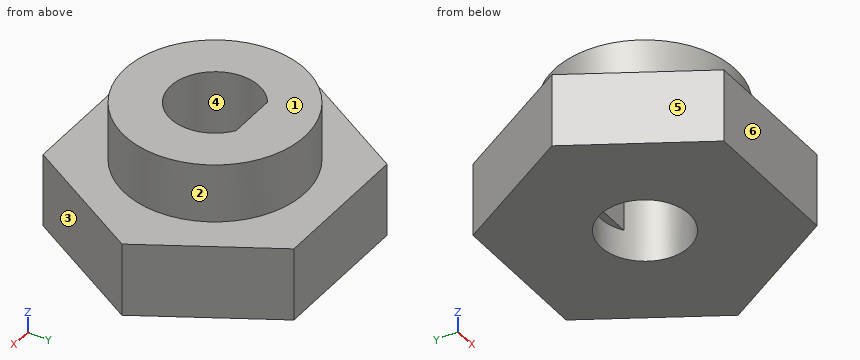
```python
from build123d import *

# Parameters (mm, degrees)
SKETCH_R      = 3
PAD_DEPTH     = 5
SKETCH001_R   = 6.1
SKETCH001_R_2 = 3
PAD001_DEPTH  = 10
PAD002_DEPTH  = 13
SKETCH003_R   = 6.1
POCKET_DEPTH  = 6


with BuildPart() as part:
    # Sketch → Pad (new body)
    with BuildSketch(Plane.XY):
        Polygon((9.814955, 0), (4.907477, 8.5), (-4.907477, 8.5), (-9.814955, 0), (-4.907477, -8.5), (4.907477, -8.5), align=None)
        Circle(SKETCH_R, mode=Mode.SUBTRACT)
    extrude(amount=PAD_DEPTH)

    # Sketch001 (on Face9 of Pad) → Pad001 (join)
    with BuildSketch(Plane.XY.offset(5)):
        Circle(SKETCH001_R)
        Circle(SKETCH001_R_2, mode=Mode.SUBTRACT)
    extrude(amount=PAD001_DEPTH)

    # Sketch002 (on Face12 of Pad001) → Pad002 (join)
    with BuildSketch(Plane.XY.offset(15)):
        with BuildLine():
            Line((-1.658312, 2.5), (1.658312, 2.5))
            ThreePointArc((1.658312, 2.5), (0, 3), (-1.658312, 2.5))
        make_face()
    extrude(amount=-PAD002_DEPTH)

    # Sketch003 (on Face15 of Pad002) → Pocket (cut)
    with BuildSketch(Plane.XY.offset(15)):
        Circle(SKETCH003_R)
    extrude(amount=-POCKET_DEPTH, mode=Mode.SUBTRACT)


solid = part.part
```
For this review, take the finished solid that the model builds, in its own axes (mm). Face numbers are marked on the shaded views. A direction names the side the tool comes from. Round coordinates to 2 decimals unless told otherwise and drop trailing zeros. Order: outer loops, then holes, each group sorted by start corner. A loop starts at its lowest first (then second) coordinate and runs counter-clockwise, first axis right, second up.
Q1. We need section D-D, the plane z = 1.5. Give the boundary of the cut face in (x, y), plus the area to 3 significant figures.
Findings below:
outline: (-9.81, 0) - (-4.91, -8.5) - (4.91, -8.5) - (9.81, 0) - (4.91, 8.5) - (-4.91, 8.5) - close; hole circle Ø6 at (0, 0)
area: 222 mm2
Q2. We need section C-C, the plane y = 2. Give the boundary of the cut face in (x, z), plus the area to 3 significant figures.
Findings below:
outline: (-8.66, 0) - (-2.24, 0) - (-2.24, 9) - (-5.76, 9) - (-5.76, 5) - (-8.66, 5) - close; (2.24, 0) - (8.66, 0) - (8.66, 5) - (5.76, 5) - (5.76, 9) - (2.24, 9) - close
area: 92.5 mm2
Q3. Machinability: for the marked faces 1 and 2, which of the approach directions +Z, -Z, +X, -X, +Y, -Y give a long, thin tool a straight path to every point of the face, cutting with its end or side? Answer none if there is none.
Findings below:
face 1: +Z, +X, -X, +Y, -Y
face 2: +Z
Q4. We need section B-B, the plane z = 4.5. Give the boundary of the cut face in (x, y), plus the area to 3 significant figures.
Findings below:
outline: (-9.81, 0) - (-4.91, -8.5) - (4.91, -8.5) - (9.81, 0) - (4.91, 8.5) - (-4.91, 8.5) - close; hole (-1.66, 2.5) arc R3 ccw (long way) to (1.66, 2.5) - close
area: 223 mm2
Q5. Mouldability with a two-part tool opening along X and no side actions: class the marked faces 3, 4, 5 and 6 as pulls with the +X half, pulls with the -X half, needs draft (parallel to the pull), parting line crosses it, or undercut.
Findings below:
face 3: pulls with the +X half
face 4: undercut
face 5: pulls with the -X half
face 6: needs draft
Q6. Insertion check: P1, Ø2, axis at x = -6, z = 7, coming from the -Y side; P2, Ø1, axis at x = 5.5, y = 5, coming from the +Z side; P3, Ø1, axis at x = -3.5, z = 7.5, coming from the +Y side; P4, Ø1.5, axis at x = -0.5, y = 1.5, coming from the -Z side. Each pin has a flat end and moves straight along its axis. Give the tip position at first contact, or say it passes through.
Findings below:
P1: stops at y = -3.49
P2: stops at z = 5
P3: stops at y = 5.31
P4: passes through
Q7. We need section A-A, the plane x = 0. Give the boundary of the cut face in (y, z), plus the area to 3 significant figures.
Findings below:
outline: (-8.5, 0) - (-3, 0) - (-3, 9) - (-6.1, 9) - (-6.1, 5) - (-8.5, 5) - close; (2.5, 2) - (3, 2) - (3, 0) - (8.5, 0) - (8.5, 5) - (6.1, 5) - (6.1, 9) - (2.5, 9) - close
area: 83.3 mm2
Q8. Wall thickness on line 1 (Y direction, x = 0, z = 5.5); line 2 (Y direction, x = 0, z = 3.75); line 3 (Z direction, x = 8, y = 0.25): over which ranges is each line inside the solid? List them lowest first.
Findings below:
line 1: y = -6.1 to -3, 2.5 to 6.1
line 2: y = -8.5 to -3, 2.5 to 8.5
line 3: z = 0 to 5
